Design review of the part built by this model. Coordinates are the model's own, in mm. Give positions to 0.01 mm unless a question says otherwise; leave off trailing zeros. Loops run counter-clockwise (first coordinate to the right, second up) from the corner with the lowest first, then second, coordinate; pieces in that order, holes last.
from build123d import *

# Parameters (mm, degrees)
SKIZZE1_W                       = 30
SKIZZE1_H                       = 6
AUFSATZ_LINEAR_AUSTRAGEN1_DEPTH = 65
CUT_EXTRUDE1_DEPTH              = 67.775744099
CUT_EXTRUDE1_DEPTH_BACK         = 67.775744099
SKETCH1_R                       = 4.5


with BuildPart() as part:
    # Skizze1 → Aufsatz-Linear austragen1 (new, symmetric)
    with BuildSketch(Plane.XY):
        Rectangle(SKIZZE1_W, SKIZZE1_H)
    extrude(amount=AUFSATZ_LINEAR_AUSTRAGEN1_DEPTH, both=True)

    # Sketch1 → Cut-Extrude1 (cut, two sides: drawn at the far end of the back side and taken through both)
    with BuildSketch(Plane(origin=(0, 0, 0), x_dir=(1, 0, 0), z_dir=(0, 1, 0)).offset(-CUT_EXTRUDE1_DEPTH_BACK)):
        with Locations(Location((8, 0, 0), (0, 0, 270))):
            Circle(SKETCH1_R)
    extrude(amount=CUT_EXTRUDE1_DEPTH + CUT_EXTRUDE1_DEPTH_BACK, mode=Mode.SUBTRACT)


solid = part.part
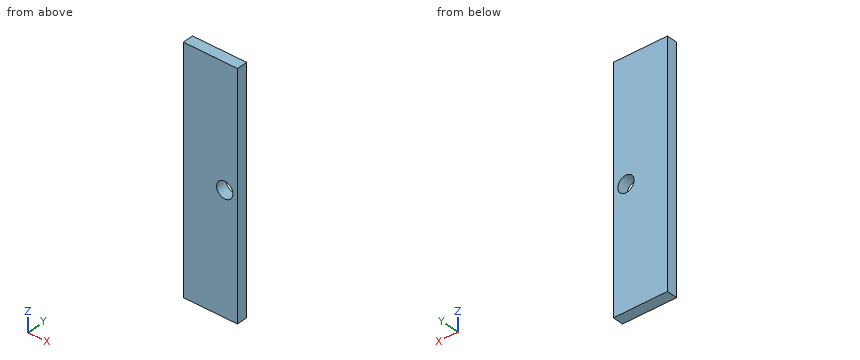
Q1. Take a section at C-C (y = 0.85). Give the boundary of the cut face in (x, z).
Results:
outline: (-15, -65) - (15, -65) - (15, 65) - (-15, 65) - close; hole circle Ø9 at (8, 0)
Q2. Take a section at A-A (z = 0). Give the boundary of the cut face in (x, y).
Results:
outline: (-15, -3) - (3.5, -3) - (3.5, 3) - (-15, 3) - close; (12.5, -3) - (15, -3) - (15, 3) - (12.5, 3) - close
Q3. Take a section at B-B (x = 8). Give the boundary of the cut face in (y, z).
Results:
outline: (-3, -65) - (3, -65) - (3, -4.5) - (-3, -4.5) - close; (-3, 4.5) - (3, 4.5) - (3, 65) - (-3, 65) - close
Q4. Insertion check: pin 1 (14.5 mm diameter, centred on x = 8, z = 0, fed in from +Y). The pin has a flat end and moves straight along its axis. Give the tip position at first contact, or say it passes through.
Results:
pin 1: stops at y = 3
Q5. Wall thickness on line 1 (X direction, y = -0.7, z = 0); line 2 (Z direction, x = 8, y = 1); line 3 (Z direction, x = 6.5, y = -0.9): over which ranges is each line inside the solid? List them lowest first.
Results:
line 1: x = -15 to 3.5, 12.5 to 15
line 2: z = -65 to -4.5, 4.5 to 65
line 3: z = -65 to -4.24, 4.24 to 65
